Geometry check sheet. Reference: the model listing, model coordinates, mm. Coordinates: 2 decimals unless noted, no trailing zeros. Write each loop counter-clockwise with the first axis right and the second up, starting at its lowest first coordinate (ties: lowest second). Pieces come first, ordered by that corner, then holes. Notation, with made-up numbers: (14, 27) - (62, 27) arc R20 cw to (62, 46) - close; hole circle Ø8 at (49.25, 4). An arc over 180 degrees is marked (long way). Answer as a JSON object with one key per item and string values. Group by question number.
from build123d import *

# Parameters (mm, degrees)
ESQUISSE1_W             = 20
ESQUISSE1_H             = 355
BOSS_EXTRU_1_DEPTH      = 11
ENL_V_MAT_EXTRU_1_DEPTH = 356.311131264
ENL_V_MAT_EXTRU_2_DEPTH = 356.311131264
ENL_V_MAT_EXTRU_3_DEPTH = 356.311131264
ENL_V_MAT_EXTRU_4_DEPTH = 356.311131264
PER_AGE1_D              = 4.917
PER_AGE1_DEPTH          = 11
PER_AGE2_D              = 4.917
CHANFREIN1_SIZE         = 0.5415
CHANFREIN2_SIZE         = 0.3


with BuildPart() as part:
    # Esquisse1 → Boss.-Extru.1 (new body)
    with BuildSketch(Plane.XZ):
        with Locations((0, 72.5)):
            Rectangle(ESQUISSE1_W, ESQUISSE1_H)
    extrude(amount=-BOSS_EXTRU_1_DEPTH)

    # Esquisse2 → Enlèv. mat.-Extru.1 (cut, through all)
    with BuildSketch(Plane(origin=(0, 0, -105), x_dir=(-1, 0, 0), z_dir=(0, 0, -1))):
        with BuildLine():
            Line((10, 7.9), (10, 10.22385))
            Line((10, 10.22385), (9.440021531, 9.900556887))
            ThreePointArc((9.440021531, 9.900556887), (9.015681976, 9.557293765), (8.71772889, 9.1))
            Line((8.71772889, 9.1), (7.5, 9.1))
            Line((7.5, 9.1), (7.5, 7.9))
            Line((7.5, 7.9), (10, 7.9))
        make_face()
    extrude(amount=-ENL_V_MAT_EXTRU_1_DEPTH, mode=Mode.SUBTRACT)

    # Esquisse3 → Enlèv. mat.-Extru.2 (cut, through all)
    with BuildSketch(Plane(origin=(0, 0, -105), x_dir=(-1, 0, 0), z_dir=(0, 0, -1))):
        with BuildLine():
            Line((9.440021531, 7.099443113), (10, 6.77615))
            Line((10, 6.77615), (10, 7.9))
            Line((10, 7.9), (8.71772889, 7.9))
            ThreePointArc((8.71772889, 7.9), (9.015681976, 7.442706235), (9.440021531, 7.099443113))
        make_face()
    extrude(amount=-ENL_V_MAT_EXTRU_2_DEPTH, mode=Mode.SUBTRACT)

    # Esquisse4 → Enlèv. mat.-Extru.3 (cut, through all)
    with BuildSketch(Plane(origin=(0, 0, -105), x_dir=(-1, 0, 0), z_dir=(0, 0, -1))):
        with BuildLine():
            Line((-10, 9.1), (-10, 6.77615))
            Line((-10, 6.77615), (-9.440021531, 7.099443113))
            ThreePointArc((-9.440021531, 7.099443113), (-9.015681976, 7.442706235), (-8.71772889, 7.9))
            Line((-8.71772889, 7.9), (-7.5, 7.9))
            Line((-7.5, 7.9), (-7.5, 9.1))
            Line((-7.5, 9.1), (-10, 9.1))
        make_face()
    extrude(amount=-ENL_V_MAT_EXTRU_3_DEPTH, mode=Mode.SUBTRACT)

    # Esquisse5 → Enlèv. mat.-Extru.4 (cut, through all)
    with BuildSketch(Plane(origin=(0, 0, -105), x_dir=(-1, 0, 0), z_dir=(0, 0, -1))):
        with BuildLine():
            Line((-9.440021531, 9.900556887), (-10, 10.22385))
            Line((-10, 10.22385), (-10, 9.1))
            Line((-10, 9.1), (-8.71772889, 9.1))
            ThreePointArc((-8.71772889, 9.1), (-9.015681976, 9.557293765), (-9.440021531, 9.900556887))
        make_face()
    extrude(amount=-ENL_V_MAT_EXTRU_4_DEPTH, mode=Mode.SUBTRACT)

    # Perçage1
    with Locations(Plane(origin=(0, 11, 0), x_dir=(1, 0, 0), z_dir=(0, 1, 0))):
        with Locations((0, -180), (0, -120), (0, 60), (0, 180)):
            Hole(PER_AGE1_D / 2, depth=PER_AGE1_DEPTH)

    # Perçage2 (through all)
    with Locations(Plane(origin=(0, 0, 0), x_dir=(-1, 0, 0), z_dir=(0, -1, 0))):
        with Locations((0, -240), (0, -60), (0, 0), (0, 120), (0, 240)):
            Hole(PER_AGE2_D / 2)

    # Chanfrein1
    chanfrein1_edges = [part.edges().sort_by_distance(p)[0] for p in [
        (-2.4585, 0, 0),
        (-2.4585, 11, 0),
        (-2.4585, 0, 60),
        (-2.4585, 11, 60),
        (-2.4585, 0, 240),
        (-2.4585, 11, 240),
        (10, 0, 72.5),
        (-10, 0, 72.5),
        (2.4585, 11, -60),
        (2.4585, 0, -60),
        (2.4585, 11, 120),
        (2.4585, 0, 120),
        (2.4585, 11, 180),
        (2.4585, 0, 180),
    ]]
    chamfer(chanfrein1_edges, length=CHANFREIN1_SIZE)

    # Chanfrein2
    chanfrein2_edges = [part.edges().sort_by_distance(p)[0] for p in [
        (10, 11, 72.5),
        (-10, 11, 72.5),
    ]]
    chamfer(chanfrein2_edges, length=CHANFREIN2_SIZE)


solid = part.part
(1) Material ranges on L1, parallel to Y at x = -8, z = -11; L2, parallel to Y at x = -8.75, z = -5; L3, parallel to X at y = 3.25, z = -60, recorded low to high. Write a range as [from, to].
(2) Draft check along X on faces 1 (the face through (10, 4, 70)), 2 (the face through (0, 11, 75)), 3 (the face through (-10, 4, 70)). Enter one of: +X half, -X half, draft (parallel to the pull), parting line (faces both ways), or undercut.
(3) Gauge pin test, flat ends, axial feed: pin 1 (3 mm diameter, centred on x = 0, z = 120, fed in from +Y); pin 2 (1.5 mm diameter, centred on y = 7, z = 66, fed in from -X); pin 3 (1.3 mm diameter, centred on y = 9, z = 63.5, fed in from +X). Record the tip position at first contact, or that the pin passes through.
(4) Section check A-A (y = 2.5). Record the cut outline in (x, z).
Conclusion:
{
 "1": {"L1": "y = [0, 7.9], [9.1, 11]", "L2": "y = [0, 7.83], [9.17, 11]", "L3": "x = [-10, -2.46], [2.46, 10]"},
 "2": {"face 1": "+X half", "face 2": "draft", "face 3": "-X half"},
 "3": {"pin 1": "passes through", "pin 2": "stops at x = -10", "pin 3": "stops at x = 9.11"},
 "4": {"outline": "(-10, -105) - (10, -105) - (10, 250) - (-10, 250) - close; hole circle Ø4.92 at (0, -60); hole circle Ø4.92 at (0, 0); hole circle Ø4.92 at (0, 60); hole circle Ø4.92 at (0, 120); hole circle Ø4.92 at (0, 180); hole circle Ø4.92 at (0, 240)"}
}
